from build123d import *

# Parameters (mm, degrees)
BOSS_EXTRUDE1_DEPTH  = 15
RIB1_REACH           = 100.995
SKETCH2_WALL_W       = 283.344562668
SKETCH2_WALL_H       = 5
M3_CLEARANCE_HOLE1_D = 3.6
CUT_EXTRUDE2_DEPTH   = 3.5
CUT_EXTRUDE3_DEPTH   = 89.932558717


with BuildPart() as part:
    # Sketch1 → Boss-Extrude1 (new, symmetric)
    with BuildSketch(Plane.XY):
        Polygon((0, 0), (0, 80), (8, 80), (8, 8), (50, 8), (50, 0), align=None)
    extrude(amount=BOSS_EXTRUDE1_DEPTH, both=True)

    # Sketch2 wall → Rib1 (add, up to next)
    with BuildSketch(Plane(origin=(29, 44, 15), x_dir=(0.503871025524, -0.863778900898, 0), z_dir=(0.863778900898, 0.503871025524, 0)), mode=Mode.PRIVATE) as rib1_sk1:
        with Locations((0, 2.5)):
            Rectangle(SKETCH2_WALL_W, SKETCH2_WALL_H)
    rib1_tool1 = extrude(rib1_sk1.sketch, amount=-RIB1_REACH, mode=Mode.PRIVATE) - part.part
    rib1 = rib1_tool1.solids().sort_by_distance((29, 44, 15))[0]
    add(rib1)

    # Mirror1: Rib1 across plane
    add(rib1.mirror(Plane.XY))

    # M3 Clearance Hole1 (through all)
    with Locations(Plane(origin=(8, 0, 0), x_dir=(0, 0, -1), z_dir=(1, 0, 0))):
        with Locations((0, 70)):
            Hole(M3_CLEARANCE_HOLE1_D / 2)

    # Sketch6 → Cut-Extrude2 (cut)
    with BuildSketch(Plane(origin=(8, 0, 0), x_dir=(0, 0, -1), z_dir=(1, 0, 0))):
        Polygon((3.637306696, 70), (1.818653348, 73.15), (-1.818653348, 73.15), (-3.637306696, 70), (-1.818653348, 66.85), (1.818653348, 66.85), align=None)
    extrude(amount=-CUT_EXTRUDE2_DEPTH, mode=Mode.SUBTRACT)

    # Sketch7 → Cut-Extrude3 (cut, through all)
    with BuildSketch(Plane(origin=(0, 8, 0), x_dir=(1, 0, 0), z_dir=(0, 1, 0))):
        with BuildLine():
            Line((39.5, 2.75), (44.5, 2.75))
            ThreePointArc((44.5, 2.75), (47.25, 0), (44.5, -2.75))
            Line((44.5, -2.75), (39.5, -2.75))
            ThreePointArc((39.5, -2.75), (36.75, 0), (39.5, 2.75))
        make_face()
    extrude(amount=-CUT_EXTRUDE3_DEPTH, mode=Mode.SUBTRACT)


solid = part.part
Work out the finished part from the listing and answer in its coordinate system (mm). A direction names the side the tool comes from. Round coordinates to 2 decimals unless told otherwise and drop trailing zeros. Order: outer loops, then holes, each group sorted by start corner. A loop starts at its lowest first (then second) coordinate and runs counter-clockwise, first axis right, second up. Notation, with made-up numbers: M -8,24.5 L 7,24.5 A30 cw 7,52.5 Z; hole C 82,-29 d4. An arc over 180 degrees is marked long. Put each result on its own line as item: value. Start each with the question number.
Q1. Section A-A, the plane z = 0 is taken. Write down the section's boundary in (x, y).
Q2. Section C-C, the plane z = 8.75 is taken. Write down the section's boundary in (x, y).
Q3. Flat-ended cylindrical pins translate along their axes: pin 1 (3 mm diameter, centred on x = 6, z = -0.5, fed in from -Y); pin 2 (12 mm diameter, centred on y = 46.5, z = -2.5, fed in from +X); pin 3 (1.5 mm diameter, centred on x = 21.5, z = 9.5, fed in from +Y); pin 4 (5 mm diameter, centred on x = 27.5, z = 9.5, fed in from +Y). Find the tip coordinate at first contact, or state that the pin passes through.
Q4. Straight lines are drawn through the part: L1, parallel to Y at x = 3.35, z = 0; L2, parallel to Z at x = 44.5, y = 14; L3, parallel to Z at x = 3, y = 70. For each, find the intervals that lie inside material, in ascending order. Write a range as [from, to].
Q5. For a pull along X with two mould halves and no side action, classify faces 6 (the flat face through (42, 4, 2.75)), 7 (the flat face through (0, 39, 0)), 8 (the flat face through (28.71, 44.5, 12.46)) as pulls with the +X half, pulls with the -X half, needs draft (parallel to the pull), parting line crosses it, or undercut.
Q6. A tool of negligible diameter and unlimited length cuts with its end or side. For faces 1 (the cylindrical face through (47.25, 4.06, -0.06)), 2 (the flat face through (28.71, 44.5, -12.46)), 3 (the flat face through (6, 73.15, 0)), 4 (the flat face through (25, 0, 0)), 5 (the flat face through (25, 32, -10)), from which of +Z, -Z, +X, -X, +Y, -Y can it reach the whole face along a straight path? Write none if from no direction.
Q7. Section B-B, the plane y = 5 is taken. Write down the section's boundary in (x, z).
Q8. Section D-D, the plane y = 41 is taken. Write down the section's boundary in (x, z), and give its area (4 significant figures).
Findings below:
1. outline: M 0,0 L 36.75,0 L 36.75,8 L 8,8 L 8,66.85 L 4.5,66.85 L 4.5,68.2 L 0,68.2 Z; M 0,71.8 L 4.5,71.8 L 4.5,73.15 L 8,73.15 L 8,80 L 0,80 Z; M 47.25,0 L 50,0 L 50,8 L 47.25,8 Z
2. outline: M 0,0 L 50,0 L 50,8 L 8,8 L 8,80 L 0,80 Z
3. pin 1: stops at y = 0
3. pin 2: stops at x = 8
3. pin 3: stops at y = 57.82
3. pin 4: stops at y = 50.77
4. L1: y = [0, 68.2], [71.8, 80]
4. L2: z = [-15, -10], [10, 15]
4. L3: z = [-15, -1.8], [1.8, 15]
5. face 6: undercut
5. face 7: pulls with the -X half
5. face 8: pulls with the +X half
6. face 1: +Y, -Y
6. face 2: +Z, -Z, +X, +Y
6. face 3: +X
6. face 4: +Z, -Z, +X, -X, -Y
6. face 5: +X, +Y
7. outline: M 0,-15 L 50,-15 L 50,15 L 0,15 Z; hole M 39.5,-2.75 L 44.5,-2.75 A2.75 ccw 44.5,2.75 L 39.5,2.75 A2.75 ccw Z
8. outline: M 0,-15 L 30.75,-15 L 30.75,-10 L 8,-10 L 8,10 L 30.75,10 L 30.75,15 L 0,15 Z
8. area: 467.5 mm^2
